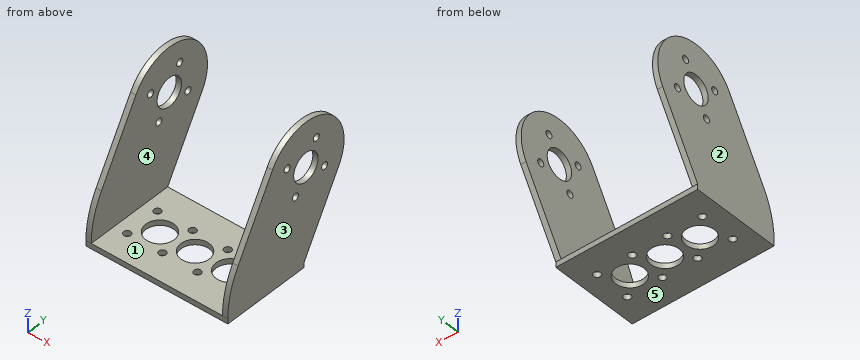
from build123d import *

# Parameters (mm, degrees)
SKETCH3_W           = 40
SKETCH3_H           = 1.5
BOSS_EXTRUDE3_DEPTH = 25
SKETCH4_R           = 4
SKETCH4_R_2         = 1
BOSS_EXTRUDE4_DEPTH = 1.5
SKETCH6_R           = 4
SKETCH6_R_2         = 1
CUT_EXTRUDE1_DEPTH  = 1.5


with BuildPart() as part:
    # Sketch3 → Boss-Extrude3 (new body)
    with BuildSketch(Plane(origin=(0, 0, 0), x_dir=(1, 0, 0), z_dir=(0, 1, 0))):
        with Locations((3.172638191, -0.75)):
            Rectangle(SKETCH3_W, SKETCH3_H)
    extrude(amount=BOSS_EXTRUDE3_DEPTH)

    # Sketch4 → Boss-Extrude4 (add)
    with BuildSketch(Plane(origin=(23.172638191, 0, 0), x_dir=(0, 0, -1), z_dir=(1, 0, 0))):
        with BuildLine():
            Line((-14, 3.349364905), (-33.522182008, 14.620501943))
            ThreePointArc((-33.522182008, 14.620501943), (-38.360080348, 31.625461179), (-21.355121112, 36.463359519))
            Line((-21.355121112, 36.463359519), (-1.5, 25))
            Line((-1.5, 25), (-1.5, 0))
            ThreePointArc((-1.5, 0), (-7.970476128, 0.851854343), (-14, 3.349364905))
        make_face()
        with Locations((-27.43865156, 25.541930731)):
            Circle(SKETCH4_R, mode=Mode.SUBTRACT)
        with Locations((-30.84502587, 19.426653627)):
            Circle(SKETCH4_R_2, mode=Mode.SUBTRACT)
        with Locations((-33.553928663, 28.948305041)):
            Circle(SKETCH4_R_2, mode=Mode.SUBTRACT)
        with Locations((-24.032277249, 31.657207834)):
            Circle(SKETCH4_R_2, mode=Mode.SUBTRACT)
        with Locations((-21.323374456, 22.13555642)):
            Circle(SKETCH4_R_2, mode=Mode.SUBTRACT)
    boss_extrude4 = extrude(amount=-BOSS_EXTRUDE4_DEPTH)

    # Mirror1: Boss-Extrude4 across plane
    add(boss_extrude4.mirror(Plane.ZY.offset(-3.172638191)))

    # Sketch6 → Cut-Extrude1 (cut)
    with BuildSketch(Plane(origin=(0, 0, 0), x_dir=(-1, 0, 0), z_dir=(0, 0, -1))):
        with Locations((-3.172638191, 12.5)):
            Circle(SKETCH6_R)
        with Locations((-13.072133128, 12.5)):
            Circle(SKETCH6_R)
        with Locations((-8.12238566, 7.550252532)):
            Circle(SKETCH6_R_2)
        with Locations((-18.021880596, 7.550252532)):
            Circle(SKETCH6_R_2)
        with Locations((-18.021880596, 17.449747468)):
            Circle(SKETCH6_R_2)
        with Locations((-8.12238566, 17.449747468)):
            Circle(SKETCH6_R_2)
        with Locations(Location((11.676604214, 17.449747468, 0), (0, 0, 180))):
            Circle(SKETCH6_R_2)
        with Locations(Location((1.777109277, 17.449747468, 0), (0, 0, 180))):
            Circle(SKETCH6_R_2)
        with Locations(Location((11.676604214, 7.550252532, 0), (0, 0, 180))):
            Circle(SKETCH6_R_2)
        with Locations(Location((6.726856745, 12.5, 0), (0, 0, 180))):
            Circle(SKETCH6_R)
        with Locations(Location((1.777109277, 7.550252532, 0), (0, 0, 180))):
            Circle(SKETCH6_R_2)
    extrude(amount=-CUT_EXTRUDE1_DEPTH, mode=Mode.SUBTRACT)


solid = part.part
Part model, mm, in its own coordinate system. Face numbers are marked on the shaded views. A direction names the side the tool comes from. Coordinates: 2 decimals unless noted, no trailing zeros. Order: outer loops, then holes, each group sorted by start corner. A loop starts at its lowest first (then second) coordinate and runs counter-clockwise, first axis right, second up. Notation, with made-up numbers: M 27,85 L 33,85 A28 ccw 33,111 Z; hole C 66,79.25 d10. An arc over 180 degrees is marked long. One line per question, with ' | ' between items.
Q1. Slice it at C-C (x = 16). Give the cut face in (y, z), and give its area (3 significant figures).
A:
outline: M 0,0 L 9.77,0 L 9.77,1.5 L 0,1.5 Z; M 15.23,0 L 25,0 L 25,1.5 L 15.23,1.5 Z | area: 29.3 mm^2
Q2. 3-axis set-ups, long thin cutter, end or side, ignore diameter. For the marked faces 4 and 5: which of +Z, -Z, +X, -X, +Y, -Y reach the whole face in a straight line?
A:
face 4: +Z, +Y, -Y | face 5: -Z, +X, -X, +Y, -Y
Q3. Slice it at B-B (y = 11). Give the cut face in (x, z), and give its area (3 significant figures).
A:
outline: M -16.83,0 L -10.43,0 L -10.43,1.5 L -15.33,1.5 L -15.33,27.25 L -16.83,27.25 Z; M -3.02,0 L -0.54,0 L -0.54,1.5 L -3.02,1.5 Z; M 6.88,0 L 9.36,0 L 9.36,1.5 L 6.88,1.5 Z; M 16.78,0 L 23.17,0 L 23.17,27.25 L 21.67,27.25 L 21.67,1.5 L 16.78,1.5 Z | area: 104 mm^2
Q4. Slice it at D-D (x = 8). Give the cut face in (y, z), and give its area (3 significant figures).
A:
outline: M 0,0 L 6.56,0 L 6.56,1.5 L 0,1.5 Z; M 8.54,0 L 16.46,0 L 16.46,1.5 L 8.54,1.5 Z; M 18.44,0 L 25,0 L 25,1.5 L 18.44,1.5 Z | area: 31.5 mm^2
Q5. Two-plate mould, pull along X, no slides. Class the marked faces 1, 2 and 3: +X half, -X half, draft (parallel to the pull), parting line (faces both ways), or undercut.
A:
face 1: undercut | face 2: -X half | face 3: +X half
Q6. Drill centre lines: line 1 (X direction, y = 32, z = 38); line 2 (Z direction, x = -9, y = 18). Where is each one in solid material? Low to high.
A:
line 1: x = -16.83 to -15.33, 21.67 to 23.17 | line 2: z = 0 to 1.5
Q7. Pin check, flat tips, straight feed: P1, Ø2.5, axis at x = 18.02, y = 7.55, coming from the +Z side; P2, Ø3, axis at y = 28.95, z = 33.55, coming from the +X side. Stop position of each tip, or through.
A:
P1: stops at z = 1.5 | P2: stops at x = 23.17
Q8. Slice it at A-A (z = 27). Give the cut face in (x, y).
A:
outline: M -16.83,10.85 L -15.33,10.85 L -15.33,21.57 L -16.83,21.57 Z; M -16.83,29.52 L -15.33,29.52 L -15.33,38.04 L -16.83,38.04 Z; M 21.67,10.85 L 23.17,10.85 L 23.17,21.57 L 21.67,21.57 Z; M 21.67,29.52 L 23.17,29.52 L 23.17,38.04 L 21.67,38.04 Z
